Geometry: final body of the model. Coordinates: model frame, mm. A direction names the side the tool comes from. Round coordinates to 2 decimals unless told otherwise and drop trailing zeros. Loops run counter-clockwise (first coordinate to the right, second up) from the corner with the lowest first, then second, coordinate; pieces in that order, holes last. Notation, with made-up numbers: (77, -2.75) - (104, -2.75) arc R11 ccw to (104, 17.25) - close; hole circle Ø1 at (-26, 21.5). An arc over 180 degrees is marked (long way). Answer as a JSON object with one key per item and string values. Group by question number.
Item 1: Section B-B (x = -0.5). Return the cut outline in (y, z).
Item 2: Reachability of faces 4 (the face through (38.47, -60, 10)), 5 (the face through (3.372, -159.746, 23.951)) from +Z, -Z, +X, -X, +Y, -Y: full face, straight path, thin tool, end or side. Return the list, or none.
Item 3: First-contact query: pin 1 (2 mm diameter, centred on y = -85, z = 24, fed in from +X); pin 2 (8 mm diameter, centred on x = 5.5, y = -16.5, fed in from -Z); pin 3 (3 mm diameter, centred on x = -1, z = 24.5, fed in from +Y). Flat tips, straight axial feed; report the tip coordinate or a pass-through.
Item 4: Draft query along Y for faces 1 (the face through (-35.19, -58, 10)), 2 (the face through (-11.011, -132.445, 24.148)), 3 (the face through (39.561, -159.746, 10.302)). Return one class per face: released by +Y, released by -Y, zero draft, split by the parting line, or undercut.
Item 5: Section D-D (y = -140). Return the cut outline in (x, z), plus the area to 3 significant figures.
Item 6: Line query: line 1 (X direction, y = 5, z = 20.75); line 2 (X direction, y = 25, z = 12.5); line 3 (Y direction, x = 6.5, z = 13.5). Output: solid intervals per line, ascending.
Item 7: Section C-C (z = 17). Return the cut outline in (x, y), plus the area to 3 significant figures.
Item 8: Section A-A (y = -107). Return the cut outline in (x, z).
```python
from build123d import *

# Parameters (mm, degrees)
F0_W     = 76.2
F0_H     = 70.9098950028
F1_DEPTH = 25.4
F2_DEPTH = 127
F3_R     = 5.08
F5_T     = -2.54
F4_W     = 21.8821829185
F4_H     = 83.6660973728
F6_DEPTH = 25.4
F7_R     = 7.62


with BuildPart() as f1:
    # F0 (on Top) → F1 (new body)
    with BuildSketch(Plane.XY):
        with Locations((2.9095611587, 1.1818297207)):
            Rectangle(F0_W, F0_H)
    extrude(amount=F1_DEPTH)

    # F2 (add): a face of the model
    f2_faces = [f1.faces().sort_by_distance(p)[0] for p in [
        (2.9095611587, -34.2731177807, 12.7),
    ]]
    extrude(f2_faces, amount=F2_DEPTH)

    # F3
    f3_edges = [f1.edges().sort_by_distance(p)[0] for p in [
        (2.909561, 36.636777, 25.4),
        (-35.190439, -62.31817, 25.4),
        (2.909561, -161.273118, 25.4),
        (41.009561, -62.31817, 25.4),
        (41.009561, -161.273118, 12.7),
        (-35.190439, -161.273118, 12.7),
    ]]
    fillet(f3_edges, radius=F3_R)

    # F5
    f5_openings = [f1.faces().sort_by_distance(p)[0] for p in [
        (2.909561, -62.246272, 0),
    ]]
    offset(amount=F5_T, openings=f5_openings)

    # F4 (on face) → F6 (cut)
    with BuildSketch(Plane(origin=(0, 0, 0), x_dir=(1, 0, 0), z_dir=(0, 0, -1))):
        with Locations((-2.2429865785, 92.903772369)):
            Rectangle(F4_W, F4_H)
    extrude(amount=-F6_DEPTH, mode=Mode.SUBTRACT)

    # F7
    f7_edges = [f1.edges().sort_by_distance(p)[0] for p in [
        (-13.184078, -134.736821, 24.13),
    ]]
    fillet(f7_edges, radius=F7_R)


solid = f1.part
```
Values:
{
 "1": {"outline": "(-161.27, 0) - (-158.73, 0) - (-158.73, 20.32) arc R2.54 cw to (-156.19, 22.86) - (-134.74, 22.86) - (-134.74, 25.4) - (-156.19, 25.4) arc R5.08 ccw to (-161.27, 20.32) - close; (-51.07, 22.86) - (31.56, 22.86) arc R2.54 cw to (34.1, 20.32) - (34.1, 0) - (36.64, 0) - (36.64, 20.32) arc R5.08 ccw to (31.56, 25.4) - (-51.07, 25.4) - close"},
 "2": {"face 4": "-Z", "face 5": "+Z, +X, -X, -Y"},
 "3": {"pin 1": "stops at x = 40.25", "pin 2": "stops at z = 22.86", "pin 3": "stops at y = 35.87"},
 "4": {"face 1": "zero draft", "face 2": "undercut", "face 3": "released by -Y"},
 "5": {"outline": "(-35.19, 0) - (-32.65, 0) - (-32.65, 20.32) arc R2.54 cw to (-30.11, 22.86) - (35.93, 22.86) arc R2.54 cw to (38.47, 20.32) - (38.47, 0) - (41.01, 0) - (41.01, 20.32) arc R5.08 ccw to (35.93, 25.4) - (-30.11, 25.4) arc R5.08 ccw to (-35.19, 20.32) - close", "area": "301 mm^2"},
 "6": {"line 1": "x = -35.17 to -32.61, 38.43 to 40.99", "line 2": "x = -35.19 to -32.65, 38.47 to 41.01", "line 3": "y = -161.27 to -158.73, 34.1 to 36.64"},
 "7": {"outline": "(-35.19, -156.19) arc R5.08 ccw to (-30.11, -161.27) - (35.93, -161.27) arc R5.08 ccw to (41.01, -156.19) - (41.01, 36.64) - (-35.19, 36.64) - close; hole (-32.65, -156.19) arc R2.54 ccw to (-30.11, -158.73) - (35.93, -158.73) arc R2.54 ccw to (38.47, -156.19) - (38.47, 34.1) - (-32.65, 34.1) - close", "area": "1,360 mm^2"},
 "8": {"outline": "(-35.19, 0) - (-32.65, 0) - (-32.65, 20.32) arc R2.54 cw to (-30.11, 22.86) - (-13.18, 22.86) - (-13.18, 25.4) - (-30.11, 25.4) arc R5.08 ccw to (-35.19, 20.32) - close; (8.7, 22.86) - (35.93, 22.86) arc R2.54 cw to (38.47, 20.32) - (38.47, 0) - (41.01, 0) - (41.01, 20.32) arc R5.08 ccw to (35.93, 25.4) - (8.7, 25.4) - close"}
}
